The drawing under review shows one solid part. Ordinate dimensions are in mm from its lowest x, y, z. A direction names the side the tool comes from. Coordinates: 2 decimals unless noted, no trailing zeros. Write each loop counter-clockwise with the first axis right and the second up, starting at its lowest first coordinate (ties: lowest second). Pieces come first, ordered by that corner, then holes.
1) Insertion check: P1, Ø1.5, axis at x = 61, y = 19.5, coming from the -Z side; P2, Ø8, axis at y = 55, z = 29, coming from the +X side; P3, Ø2, axis at x = 71, z = 19.5, coming from the +Y side; P4, Ø8, axis at x = 69.5, y = 47.5, coming from the +Z side. Each pin has a flat end and moves straight along its axis. Give the tip position at first contact, or say it passes through.
2) We need section C-C on y = 47. Write out the cut boundary in (x, z) (1 decimal), then the cut area to 3 significant figures.
3) We need section A-A on x = 46. Write out the cut boundary in (y, z) (1 decimal), then the cut area to 3 significant figures.
4) We need section B-B on z = 11.5. Write out the cut boundary in (x, y).
5) Mouldability with a two-part tool opening along X and no side actions: class the marked faces 1, 2 and 3 as pulls with the +X half, pulls with the -X half, needs draft (parallel to the pull), parting line crosses it, or undercut.
6) For the marked faces 4 and 5, list the 3-axis set-ups (+Z, -Z, +X, -X, +Y, -Y) from which the entire face can be reached by the end or side of a thin tool; tool diameter is ignored.
7) We need section D-D on z = 26. Write out the cut boundary in (x, y) (1 decimal), then the cut area to 3 significant figures.
8) To check wall thickness, follow line 1 along Y through (x, z) = (63, 16); line 2 along Z through (x, y) = (42.5, 72) (1 decimal); line 3 along X through (y, z) = (64.5, 26) (1 decimal). State the ranges of each line that lie inside material, in increasing order.
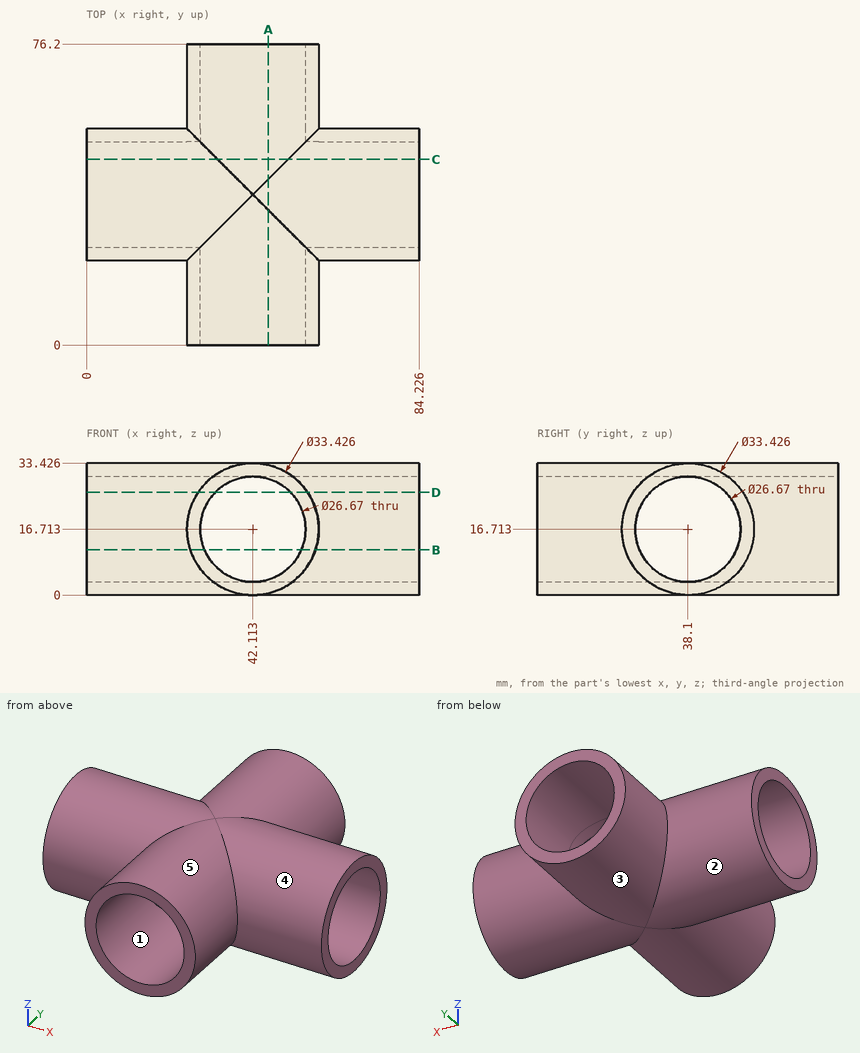
Result:
1. P1: passes through
1. P2: stops at x = 56.63
1. P3: stops at y = 54.72
1. P4: stops at z = 32.53
2. outline: (0, 2.6) - (33.2, 2.6) arc R16.7 ccw to (51, 2.6) - (84.2, 2.6) - (84.2, 6.8) - (51, 6.8) arc R13.3 cw to (33.2, 6.8) - (0, 6.8) - close; (0, 26.6) - (33.2, 26.6) arc R13.3 cw to (51, 26.6) - (84.2, 26.6) - (84.2, 30.9) - (51, 30.9) arc R16.7 ccw to (33.2, 30.9) - (0, 30.9) - close
2. area: 689 mm2
3. outline: (0, 0.5) - (34.2, 0.5) arc R16.7 ccw to (42, 0.5) - (76.2, 0.5) - (76.2, 4) - (42, 4) arc R13.3 cw to (34.2, 4) - (0, 4) - close; (0, 29.5) - (34.2, 29.5) arc R13.3 cw to (42, 29.5) - (76.2, 29.5) - (76.2, 33) - (42, 33) arc R16.7 ccw to (34.2, 33) - (0, 33) - close
3. area: 532 mm2
4. outline: (0, 22.22) - (26.23, 22.22) - (26.23, 0) - (29.84, 0) - (29.84, 25.83) - (0, 25.83) - close; (0, 50.37) - (29.84, 50.37) - (29.84, 76.2) - (26.23, 76.2) - (26.23, 53.98) - (0, 53.98) - close; (54.39, 0) - (57.99, 0) - (57.99, 22.22) - (84.23, 22.22) - (84.23, 25.83) - (54.39, 25.83) - close; (54.39, 50.37) - (84.23, 50.37) - (84.23, 53.98) - (57.99, 53.98) - (57.99, 76.2) - (54.39, 76.2) - close
5. face 1: undercut
5. face 2: needs draft
5. face 3: parting line crosses it
6. face 4: +X
6. face 5: -Y
7. outline: (0, 24.2) - (28.2, 24.2) - (28.2, 0) - (32.5, 0) - (32.5, 28.5) - (0, 28.5) - close; (0, 47.7) - (32.5, 47.7) - (32.5, 76.2) - (28.2, 76.2) - (28.2, 52) - (0, 52) - close; (51.7, 0) - (56, 0) - (56, 24.2) - (84.2, 24.2) - (84.2, 28.5) - (51.7, 28.5) - close; (51.7, 47.7) - (84.2, 47.7) - (84.2, 52) - (56, 52) - (56, 76.2) - (51.7, 76.2) - close
7. area: 982 mm2
8. line 1: y = 21.4 to 24.78, 51.42 to 54.8
8. line 2: z = 0 to 3.4, 30 to 33.4
8. line 3: x = 28.2 to 32.5, 51.7 to 56
